from build123d import *

# Parameters (mm, degrees)
SKETCH1_R           = 3.175
BOSS_EXTRUDE1_DEPTH = 12.7
SKETCH2_R           = 3.175
BOSS_EXTRUDE2_DEPTH = 4.7625
SKETCH3_W           = 1.5875
SKETCH3_H           = 0.79375
CUT_EXTRUDE1_DEPTH  = 9.525


with BuildPart() as part:
    # Sketch1 → Boss-Extrude1 (new body)
    with BuildSketch(Plane.XY):
        with BuildLine():
            Line((0, 0), (0, 19.05))
            Line((0, 19.05), (-12.7, 19.05))
            Line((-12.7, 19.05), (-12.7, 19.84375))
            Line((-12.7, 19.84375), (-0.79375, 31.75))
            Line((-0.79375, 31.75), (11.90625, 31.75))
            Line((11.90625, 31.75), (11.90625, 0))
            ThreePointArc((11.90625, 0), (5.953125, -5.953125), (0, 0))
        make_face()
        with Locations((5.953125, 0)):
            Circle(SKETCH1_R, mode=Mode.SUBTRACT)
    extrude(amount=BOSS_EXTRUDE1_DEPTH)

    # Sketch2 → Boss-Extrude2 (add)
    with BuildSketch(Plane(origin=(0, 0, 0), x_dir=(-1, 0, 0), z_dir=(0, 0, -1))):
        with Locations((-5.55625, 25.4)):
            Circle(SKETCH2_R)
    extrude(amount=BOSS_EXTRUDE2_DEPTH)

    # Sketch3 → Cut-Extrude1 (cut)
    with BuildSketch(Plane(origin=(-12.16693903, 12.16693903, 0), x_dir=(0, 0, 1), z_dir=(-0.707106781, 0.707106781, 0))):
        with Locations((-2.38125, 24.667499295)):
            Rectangle(SKETCH3_W, SKETCH3_H)
    extrude(amount=-CUT_EXTRUDE1_DEPTH, mode=Mode.SUBTRACT)


solid = part.part
Can you work these out from the model? Positions are in its coordinate system, mm. A direction names the side the tool comes from. Coordinates: 2 decimals unless noted, no trailing zeros. Write each loop counter-clockwise with the first axis right and the second up, starting at its lowest first coordinate (ties: lowest second). Pieces come first, ordered by that corner, then holes.
Q1. Imagine slicing it at D-D, the plane z = -1. List the corners of the cut face in (x, y) for me (3 decimals), plus the area to 3 significant figures.
Results found:
outline: circle Ø6.35 at (5.556, 25.4)
area: 31.7 mm2
Q2. Imagine slicing it at A-A, the plane z = 8. List the corners of the cut face in (x, y) for me (3 decimals), plus the area to 3 significant figures.
Results found:
outline: (-12.7, 19.05) - (0, 19.05) - (0, 0) arc R5.953 ccw to (11.906, 0) - (11.906, 31.75) - (-0.794, 31.75) - (-12.7, 19.844) - close; hole circle Ø6.35 at (5.953, 0)
area: 492 mm2
Q3. Imagine slicing it at C-C, the plane x = 4.5. List the corners of the cut face in (y, z) for me, plus the area to 3 significant figures.
Results found:
outline: (-5.77, 0) - (-2.82, 0) - (-2.82, 12.7) - (-5.77, 12.7) - close; (2.82, 0) - (22.41, 0) - (22.41, -4.76) - (28.39, -4.76) - (28.39, 0) - (31.75, 0) - (31.75, 12.7) - (2.82, 12.7) - close
area: 433 mm2
Q4. Which directions (+Z, -Z, +X, -X, +Y, -Y) give clear straight access to the entire face, cutting with the end or side of a thin tool? Please do faces 4 (the face through (4.091, 22.583, -2.348)), 5 (the face through (7.4, 27.3, -3.175)), 6 (the face through (0, 9, 6)).
Results found:
face 4: -Z
face 5: +X, +Y
face 6: +Z, -Z, -X, -Y
Q5. For P1, Ø4, axis at y = 14, z = 6, coming from the -X side; P2, Ø5, axis at x = -2, z = 4, coming from the -Y side; P3, Ø8.5, axis at x = 5.95, y = 0, coming from the -Z side, each with a flat end and sliding along its axis, tell me the tip position at first contact or that it passes through.
Results found:
P1: stops at x = 0
P2: stops at y = -2.39
P3: stops at z = 0
Q6. Imagine slicing it at B-B, the plane y = -0.5. List the corners of the cut face in (x, z) for me.
Results found:
outline: (0.02, 0) - (2.82, 0) - (2.82, 12.7) - (0.02, 12.7) - close; (9.09, 0) - (11.89, 0) - (11.89, 12.7) - (9.09, 12.7) - close
Q7. If we mould it in two halves opening along Z, with no side actions, what happens to faces 1 (the face through (11.906, 16, 6)), 2 (the face through (5, 17, 0)), 3 (the face through (7.4, 27.3, -1.588))? For each: +Z half, -Z half, draft (parallel to the pull), parting line (faces both ways), or undercut.
Results found:
face 1: draft
face 2: -Z half
face 3: undercut
Q8. Please list where these lines run through material, in increasing order: L1, parallel to Z at x = 10.25, y = 23.5; L2, parallel to Y at x = 5, z = 5; L3, parallel to Y at x = 8, z = 2.25.
Results found:
L1: z = 0 to 12.7
L2: y = -5.88 to -3.03, 3.03 to 31.75
L3: y = -5.59 to -2.43, 2.43 to 31.75
